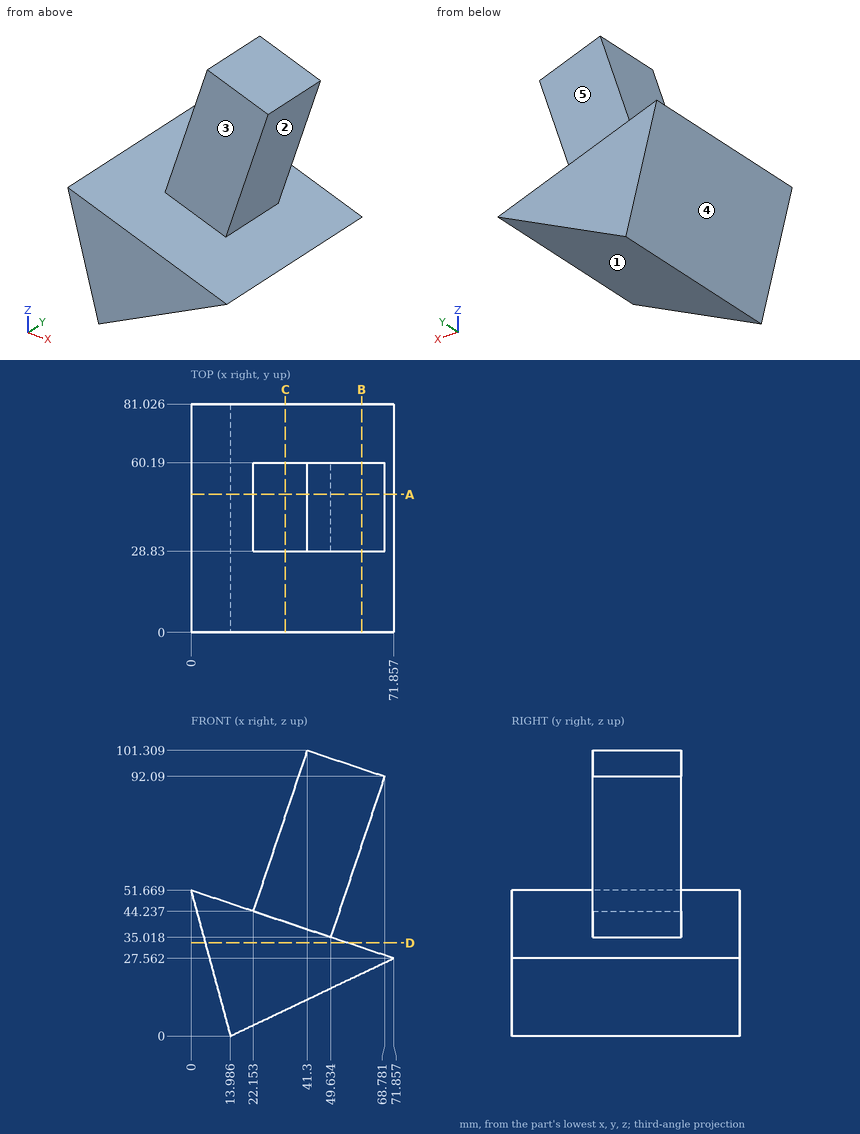
Drawing for the job (mm, zero at the part's lowest x, y, z). A direction names the side the tool comes from. Give positions to 0.01 mm unless a question says otherwise; leave off trailing zeros. Write each loop counter-clockwise with the first axis right and the second up, starting at its lowest first coordinate (ties: lowest second). Pieces come first, ordered by that corner, then holes. Notation, with made-up numbers: M 81.5,4.5 L 137.5,4.5 A8 ccw 137.5,9.5 Z; hole C 37,-2 d3. An arc over 180 degrees is marked long. Return JSON: item names as keys, results as strings. Group by question number.
(1) Mould opens along Z. For the marked faces 1, 2 and 3 say: pulls with the +Z half, pulls with the -Z half, needs draft (parallel to the pull), parting line crosses it, or undercut.
(2) Band-saw the part on B-B (x = 60.5). Give the cut face in (y, z), and give its area (3 significant figures).
(3) Drill centre lines: L1, parallel to Y at x = 43.5, z = 44.5; L2, parallel to Z at x = 31.5, y = 28; L3, parallel to X at y = 49.5, z = 80.5. Where is each one in solid material? Low to high. Write a range as [from, to].
(4) Band-saw the part on D-D (z = 33). Give the cut face in (x, y), and give its area (3 significant figures).
(5) Band-saw the part on C-C (x = 33.5). Give the cut face in (y, z).
(6) Band-saw the part on A-A (y = 49). Give the cut face in (x, z) (1 decimal).
(7) 3-axis set-ups, long thin cutter, end or side, ignore diameter. For the marked faces 4 and 5: which of +Z, -Z, +X, -X, +Y, -Y reach the whole face in a straight line?
(8) Flat gauge pins, fed straight in: pin 1 Ø3 at (x, y) = (55, 39.5) entering from -Z; pin 2 Ø5 at (y, z) = (49, 34) entering from -X; pin 3 Ø6 at (x, y) = (48, 66) entering from -Z; pin 4 Ø1 at (x, z) = (7.5, 31.5) entering from -Y. Where does each tip first touch, or does it go through?
Entries:
{
 "1": {"face 1": "pulls with the -Z half", "face 2": "undercut", "face 3": "needs draft"},
 "2": {"outline": "M 0,22.15 L 81.03,22.15 L 81.03,31.37 L 0,31.37 Z; M 28.83,67.41 L 60.19,67.41 L 60.19,94.87 L 28.83,94.87 Z", "area": "1,610 mm^2"},
 "3": {"L1": "y = [28.83, 60.19]", "L2": "z = [8.34, 41.1]", "L3": "x = [34.32, 64.89]"},
 "4": {"outline": "M 5.05,0 L 55.65,0 L 55.65,81.03 L 5.05,81.03 Z", "area": "4,100 mm^2"},
 "5": {"outline": "M 0,9.29 L 81.03,9.29 L 81.03,40.43 L 60.19,40.43 L 60.19,78.06 L 28.83,78.06 L 28.83,40.43 L 0,40.43 Z"},
 "6": {"outline": "M 0,51.7 L 14,0 L 71.9,27.6 L 49.6,35 L 68.8,92.1 L 41.3,101.3 L 22.2,44.2 Z"},
 "7": {"face 4": "-Z, -X, +Y, -Y", "face 5": "+Z, +X, +Y"},
 "8": {"pin 1": "stops at z = 18.82", "pin 2": "stops at x = 4.11", "pin 3": "stops at z = 14.77", "pin 4": "stops at y = 0"}
}
